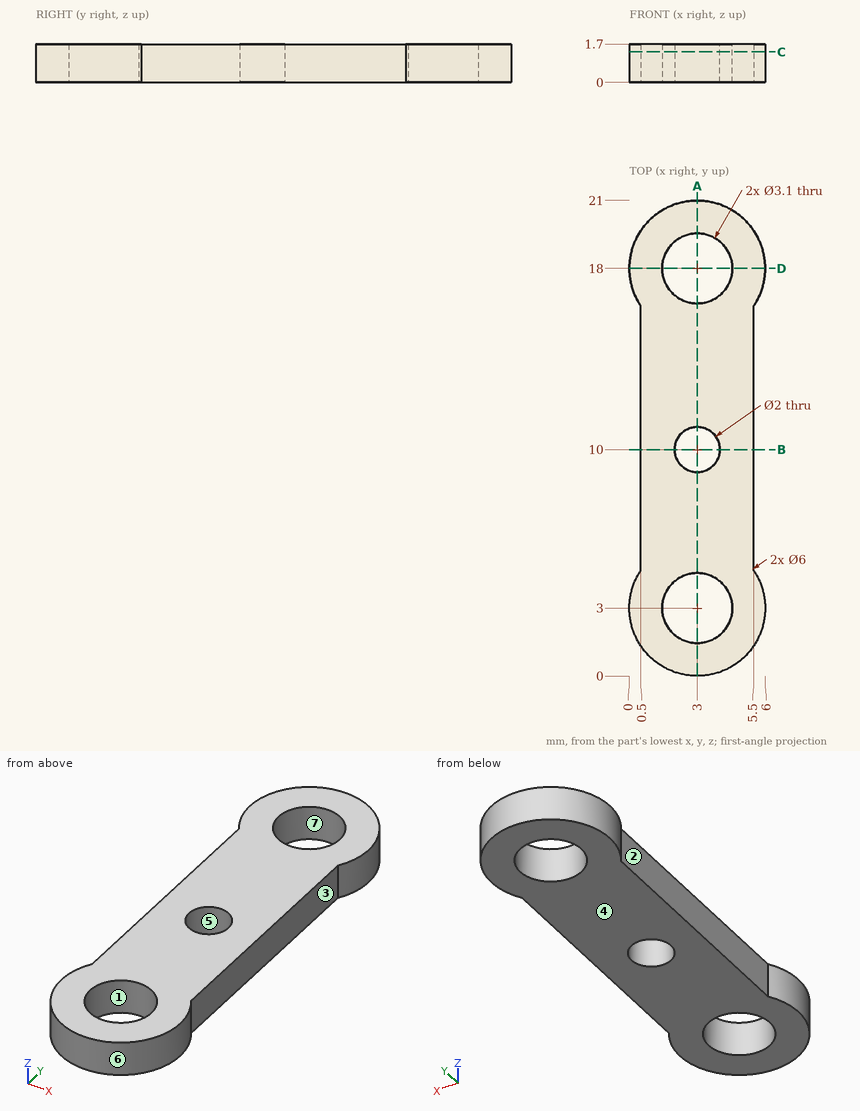
Part print with two shaded views. Sizes in mm from the minimum x, y, z corner. A direction names the side the tool comes from. Round coordinates to 2 decimals unless told otherwise and drop trailing zeros. Loops run counter-clockwise (first coordinate to the right, second up) from the corner with the lowest first, then second, coordinate; pieces in that order, holes last. Notation, with made-up numbers: M 49.5,36 L 53.5,36 A14 ccw 53.5,50 Z; hole C -1,15 d2. An arc over 180 degrees is marked long. Return JSON: item names as keys, results as strings. Group by question number.
(1) Saw through at B-B, the plane y = 10. List the corners of the cut face in (x, z).
(2) Mould opens along X. For the marked faces 4, 5, 6 and 7 say: +X half, -X half, draft (parallel to the pull), parting line (faces both ways), or undercut.
(3) Tool access for the marked faces 1, 2 and 3: list every direction of +Z, -Z, +X, -X, +Y, -Y with a clear straight run to the whole face (end or side of a thin tool).
(4) Saw through at A-A, the plane x = 3. List the corners of the cut face in (y, z), and give its area (3 significant figures).
(5) Wall check: probe 1 along Y at (x, z) = (2.9, 1.5); probe 2 along X at (y, z) = (18, 0.9); probe 3 along Y at (x, z) = (3.75, 0.55). Give the ranges that are in metal, low to high. Write a range as [from, to].
(6) Saw through at D-D, the plane y = 18. List the corners of the cut face in (x, z), and give its area (3 significant figures).
(7) Saw through at C-C, the plane z = 1.35. List the corners of the cut face in (x, y).
(8) Drop flat-ended pins along their axis: P1, Ø1, axis at x = 4.5, z = 0, coming from the +Y side; P2, Ø1.8, axis at x = 3, y = 10, coming from the +Z side; P3, Ø0.8, axis at y = 7.5, z = 1, coming from the -X side. Give the stop position or say it passes through.
Answer list:
{
 "1": {"outline": "M 0.5,0 L 2,0 L 2,1.7 L 0.5,1.7 Z; M 4,0 L 5.5,0 L 5.5,1.7 L 4,1.7 Z"},
 "2": {"face 4": "draft", "face 5": "undercut", "face 6": "parting line", "face 7": "undercut"},
 "3": {"face 1": "+Z, -Z", "face 2": "+Z, -Z, -X", "face 3": "+Z, -Z, +X"},
 "4": {"outline": "M 0,0 L 1.45,0 L 1.45,1.7 L 0,1.7 Z; M 4.55,0 L 9,0 L 9,1.7 L 4.55,1.7 Z; M 11,0 L 16.45,0 L 16.45,1.7 L 11,1.7 Z; M 19.55,0 L 21,0 L 21,1.7 L 19.55,1.7 Z", "area": "21.8 mm2"},
 "5": {"probe 1": "[0, 1.45], [4.55, 9.01], [10.99, 16.45], [19.55, 21]", "probe 2": "[0, 1.45], [4.55, 6]", "probe 3": "[0.1, 1.64], [4.36, 9.34], [10.66, 16.64], [19.36, 20.9]"},
 "6": {"outline": "M 0,0 L 1.45,0 L 1.45,1.7 L 0,1.7 Z; M 4.55,0 L 6,0 L 6,1.7 L 4.55,1.7 Z", "area": "4.93 mm2"},
 "7": {"outline": "M 0.5,4.66 A3 ccw long 5.5,4.66 L 5.5,16.34 A3 ccw long 0.5,16.34 Z; hole C 3,3 d3.1; hole C 3,18 d3.1; hole C 3,10 d2"},
 "8": {"P1": "y = 20.83", "P2": "through", "P3": "x = 0.5"}
}
